```python
from build123d import *

# Parameters (mm, degrees)
FILLET1_R                = 2.5
CIRPATTERN3_COUNT        = 4
FILLET1_OF_CIRPATTERN3_R = 2.5
SKETCH3_W                = 9
SKETCH3_H                = 9
CUT_EXTRUDE1_DEPTH       = 11


with BuildPart() as part:
    # Sketch1 → Revolve1 (revolve)
    with BuildSketch(Plane.XY, mode=Mode.PRIVATE) as revolve1_sk:
        with BuildLine():
            Line((0, 7.830238727), (0, -8.169761273))
            Line((0, -8.169761273), (-9.68857754, -8.169761273))
            ThreePointArc((-9.68857754, -8.169761273), (-12, -0.169761273), (-9.68857754, 7.830238727))
            Line((-9.68857754, 7.830238727), (0, 7.830238727))
        make_face()
    revolve(revolve1_sk.sketch.rotate(Axis((0, 7.830238727, 0), (0, -1, 0)), 270), axis=Axis((0, 7.830238727, 0), (0, -1, 0)))

    # Sketch2 → Revolve2 (revolve)
    with BuildSketch(Plane.XY):
        with BuildLine():
            Line((0, 0), (-35, 0))
            ThreePointArc((-35, 0), (-32.975720289, -4.493734325), (-28.26878394, -5.95527691))
            Line((-28.26878394, -5.95527691), (0, -2.484306687))
            Line((0, -2.484306687), (0, 0))
        make_face()
    revolve2 = revolve(axis=Axis((0, 0, 0), (-1, 0, 0)))

    # Fillet1
    fillet1_edges = [part.edges().sort_by_distance(p)[0] for p in [
        (-11.440440634, 3.889016163, 1e-09),
    ]]
    fillet(fillet1_edges, radius=FILLET1_R)

    # CirPattern3: Revolve2 ×4 about axis
    cirpattern3_axis = Axis((0, 7.830238727, 0), (0, 1, 0))
    for i in range(1, CIRPATTERN3_COUNT):
        add(revolve2.rotate(cirpattern3_axis, i * 360 / CIRPATTERN3_COUNT))

    # Fillet1 of CirPattern3
    fillet1_of_cirpattern3_edges = [part.edges().sort_by_distance(p)[0] for p in [
        (1e-09, 3.889016163, 11.440440634),
        (11.440440634, 3.889016163, -1e-09),
        (-1e-09, 3.889016163, -11.440440634),
    ]]
    fillet(fillet1_of_cirpattern3_edges, radius=FILLET1_OF_CIRPATTERN3_R)

    # Sketch3 → Cut-Extrude1 (cut)
    with BuildSketch(Plane(origin=(0, 7.830238727, 0), x_dir=(1, 0, 0), z_dir=(0, 1, 0))):
        Rectangle(SKETCH3_W, SKETCH3_H)
    extrude(amount=-CUT_EXTRUDE1_DEPTH, mode=Mode.SUBTRACT)


solid = part.part
```
Can you work these out from the model? Positions are in its coordinate system, mm. A direction names the side the tool comes from. Round coordinates to 2 decimals unless told otherwise and drop trailing zeros. Loops run counter-clockwise (first coordinate to the right, second up) from the corner with the lowest first, then second, coordinate; pieces in that order, holes last. Notation, with made-up numbers: M -10,7 L 15,7 A22 ccw 15,37 Z; hole C 72,26 d11. An arc over 180 degrees is marked long. Answer in a Markdown table with one row per item.
1. On a 3-axis mill with a long thin cutter (end or side, diameter ignored), from which of +Z, -Z, +X, -X, +Y, -Y can I reach the whole of each face in a straight line? I mean faces 4 (the face through (20.636, 0.653, -4.975)), 5 (the face through (-4.5, 2, 0)), 6 (the face through (0, -8.17, 0)). Say none if no direction works.
Established:
| item | result |
|---|---|
| face 4 | none |
| face 5 | +Y |
| face 6 | +Z, -Z, +X, -X, -Y |
2. I'm going to push flat-ended pins straight in: pin 1 Ø2 at (x, y) = (0, 1.5) entering from -Z; pin 2 Ø1.5 at (x, y) = (3, -4.5) entering from +Z; pin 3 Ø3 at (x, y) = (24.5, 0) entering from +Z. Where does each tip first touch, or does it pass through?
Established:
| item | result |
|---|---|
| pin 1 | z = -34.98 |
| pin 2 | z = 32.78 |
| pin 3 | z = 5.68 |
3. Thinking about a two-plate mould opening in X: for faces 1 (the face through (6, 7.83, 0)), 2 (the face through (0, 2, 4.5)), 3 (the face through (-1.507, -4.786, -20.634)), which applies, pulls with the +X half, pulls with the -X half, needs draft (parallel to the pull), parting line crosses it, or undercut?
Established:
| item | result |
|---|---|
| face 1 | needs draft |
| face 2 | undercut |
| face 3 | parting line crosses it |
4. If we section it at B-B, the plane x = 15.5: Please give me the cut outline in (y, z), plus the area to 3 significant figures.
Established:
| item | result |
|---|---|
| outline | C 0,0 d8.77 |
| area | 60.5 mm² |
5. Please list where these lines run through material, in increasing order: line 1 (X direction, y = -1.25, z = 3); line 2 (Y direction, x = 0.5, z = -28.5); line 3 (Z direction, x = 24.5, y = 3.5). Write a range as from..to.
Established:
| item | result |
|---|---|
| line 1 | -34.04..-4.5, 4.5..34.04 |
| line 2 | -5.96..5.96 |
| line 3 | -4.23..4.23 |
6. If we section it at A-A, the plane x = -26: Please give me the cut outline in (y, z).
Established:
| item | result |
|---|---|
| outline | C 0,0 d11.35 |
